Geometry check sheet. Reference: the model listing, model coordinates, mm. Face numbers are marked on the shaded views. A direction names the side the tool comes from. Round coordinates to 2 decimals unless told otherwise and drop trailing zeros. Order: outer loops, then holes, each group sorted by start corner. A loop starts at its lowest first (then second) coordinate and runs counter-clockwise, first axis right, second up. Notation, with made-up numbers: M 47,56 L 63,56 A19 cw 63,79 Z; hole C 66,46.5 d5. An arc over 180 degrees is marked long. Return JSON: item names as keys, results as strings. Group by question number.
```python
from build123d import *

# Parameters (mm, degrees)
CROQUIS1_R                   = 25
SALIENTE_EXTRUIR1_DEPTH      = 20
KEYWAY_DEPTH                 = 21
TALADRO_DE_MARGEN_PARA_M41_D = 4.3


with BuildPart() as part:
    # Croquis1 → Saliente-Extruir1 (new body)
    with BuildSketch(Plane.XY):
        Circle(CROQUIS1_R)
    extrude(amount=SALIENTE_EXTRUIR1_DEPTH)

    # KeySketch → Keyway (cut, through all)
    with BuildSketch(Plane(origin=(-0.358560603, -1.171254478, 20), x_dir=(1, 0, 0), z_dir=(0, 0, 1))):
        with BuildLine():
            Line((-3.641439397, 13.540571355), (-3.641439397, 17.471254478))
            Line((-3.641439397, 17.471254478), (4.358560603, 17.471254478))
            Line((4.358560603, 17.471254478), (4.358560603, 13.540571355))
            ThreePointArc((4.358560603, 13.540571355), (0.358560603, -11.828745522), (-3.641439397, 13.540571355))
        make_face()
    extrude(amount=-KEYWAY_DEPTH, mode=Mode.SUBTRACT)

    # Taladro de margen para M41 (through all)
    with Locations(Plane.XY.offset(20)):
        with Locations((21, 0), (10.5, -18.186533479), (-10.5, -18.186533479), (-21, 0), (-10.5, 18.186533479), (10.5, 18.186533479)):
            Hole(TALADRO_DE_MARGEN_PARA_M41_D / 2)


solid = part.part
```
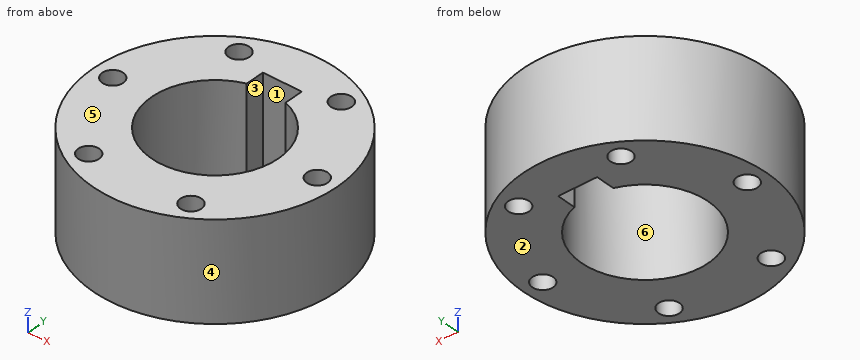
Q1. Section check A-A on x = 0. Record the cut outline in (y, z), plus the area to 3 significant figures.
Q2. Section check D-D on z = 18.75. Record the cut outline in (x, y).
Q3. Material ranges on line 1 along X through (y, z) = (17.5, 8); line 2 along Y through (x, z) = (10.5, 8.5); line 3 along Y through (x, z) = (0, 12), recorded low to high.
Q4. Depth check by flat-ended pin: pin 1 Ø1 at (x, z) = (16, 13) entering from -Y; pin 2 Ø9 at (x, z) = (-1.5, 14.5) entering from -Y; pin 3 Ø4.5 at (y, z) = (13.5, 5) entering from +X; pin 4 Ø5.5 at (x, y) = (-10.5, -18.19) entering from -Z. Enter the tip coordinate at first touch or a pass-through.
Q5. Section check B-B on y = 0. Record the cut outline in (x, z), plus the area to 3 significant figures.
Q6. Set-up check for the marked faces 1 and 2: record each of +Z, -Z, +X, -X, +Y, -Y from which the full face is reachable in a straight line by a thin tool's end or side.
Q7. Release check for a two-part mould opening along X. For the marked faces 3, 4, 5 and 6 record: +X half, -X half, draft (parallel to the pull), parting line (faces both ways), or undercut.
Q8. Section check C-C on y = -5. Record the cut outline in (x, z), plus the area to 3 significant figures.
Geometry check:
{
 "1": {"outline": "M -25,0 L -13,0 L -13,20 L -25,20 Z; M 16.3,0 L 25,0 L 25,20 L 16.3,20 Z", "area": "414 mm^2"},
 "2": {"outline": "C 0,0 d50; hole C -21,0 d4.3; hole C -10.5,-18.19 d4.3; hole C -10.5,18.19 d4.3; hole M -4,12.37 A13 ccw long 4,12.37 L 4,16.3 L -4,16.3 Z; hole C 10.5,-18.19 d4.3; hole C 10.5,18.19 d4.3; hole C 21,0 d4.3"},
 "3": {"line 1": "x = -17.85 to -12.54, -8.46 to 8.46, 12.54 to 17.85", "line 2": "y = -22.69 to -20.34, -16.04 to -7.66, 7.66 to 16.04, 20.34 to 22.69", "line 3": "y = -25 to -13, 16.3 to 25"},
 "4": {"pin 1": "stops at y = -19.62", "pin 2": "stops at y = -25", "pin 3": "stops at x = 22.33", "pin 4": "stops at z = 0"},
 "5": {"outline": "M -25,0 L -23.15,0 L -23.15,20 L -25,20 Z; M -18.85,0 L -13,0 L -13,20 L -18.85,20 Z; M 13,0 L 18.85,0 L 18.85,20 L 13,20 Z; M 23.15,0 L 25,0 L 25,20 L 23.15,20 Z", "area": "308 mm^2"},
 "6": {"face 1": "+Z, -Z", "face 2": "-Z, +X, -X, +Y, -Y"},
 "7": {"face 3": "undercut", "face 4": "parting line", "face 5": "draft", "face 6": "undercut"},
 "8": {"outline": "M -24.49,0 L -12,0 L -12,20 L -24.49,20 Z; M 12,0 L 24.49,0 L 24.49,20 L 12,20 Z", "area": "500 mm^2"}
}
